Read the model definition and answer for the solid it produces. Units are mm, in the model's axes. Face numbers are marked on the shaded views. A direction names the side the tool comes from. Coordinates: 2 decimals unless noted, no trailing zeros. Write each loop counter-clockwise with the first axis right and the second up, starting at its lowest first coordinate (ties: lowest second). Pieces come first, ordered by that corner, then holes. Notation, with made-up numbers: (41.5, 55.25) -> (84.5, 55.25) arc R25 ccw to (84.5, 88.25) -> close; hole circle Ø8 at (62.25, 55). An arc over 180 degrees is marked (long way). Answer as a JSON object with one key per item and string values. Group by question number.
(1) Find section D-D (y = 38.1). Give the vertices of the cut face in (x, z).
(2) Find section B-B (x = 42.5). Give the vertices of the cut face in (y, z), then the cut area to 3 significant figures.
(3) For a pull along Z with two mould halves and no side action, classify the marked faces 1, 2, 3 and 4 as +Z half, -Z half, draft (parallel to the pull), parting line (faces both ways), or undercut.
(4) Straight lines are drawn through the part: L1, parallel to Y at x = 72, z = -25; L2, parallel to Z at x = 69, y = 38; L3, parallel to Y at x = 38.5, z = -17. For each, find the intervals that lie inside material, in ascending order.
(5) Which of the six approach directions +Z, -Z, +X, -X, +Y, -Y give full straight-line access (tool end or side, diameter ignored) to the marked faces 5 and 6?
(6) Find section C-C (z = -28). Give the vertices of the cut face in (x, y), then the cut area to 3 significant figures.
(7) Flat-ended cylindrical pins translate along their axes: P1, Ø12.5, axis at x = 28, z = -26.5, coming from the +Y side; P2, Ø23, axis at y = 38.1, z = -25.4, coming from the +X side. Find the tip coordinate at first contact, or state that the pin passes through.
(8) Find section A-A (y = 54). Give the vertices of the cut face in (x, z).
from build123d import *

# Parameters (mm, degrees)
SKETCH1_W           = 76.2
SKETCH1_H           = 50.8
BOSS_EXTRUDE1_DEPTH = 76.2
SKETCH2_W           = 38.1
SKETCH2_H           = 25.4
CUT_EXTRUDE1_DEPTH  = 25.4
SKETCH3_R           = 12.7
CUT_EXTRUDE3_DEPTH  = 12.7


with BuildPart() as part:
    # Sketch1 → Boss-Extrude1 (new body)
    with BuildSketch(Plane(origin=(0, 0, 0), x_dir=(1, 0, 0), z_dir=(0, 1, 0))):
        with Locations((38.1, 25.4)):
            Rectangle(SKETCH1_W, SKETCH1_H)
    extrude(amount=BOSS_EXTRUDE1_DEPTH)

    # Sketch2 → Cut-Extrude1 (cut)
    with BuildSketch(Plane(origin=(0, 76.2, 0), x_dir=(1, 0, 0), z_dir=(0, 1, 0))):
        with Locations((31.75, 25.4)):
            Rectangle(SKETCH2_W, SKETCH2_H)
    extrude(amount=-CUT_EXTRUDE1_DEPTH, mode=Mode.SUBTRACT)

    # Sketch3 → Cut-Extrude3 (cut)
    with BuildSketch(Plane(origin=(76.2, 0, 0), x_dir=(0, 0, -1), z_dir=(1, 0, 0))):
        with Locations((25.4, 38.1)):
            Circle(SKETCH3_R)
    extrude(amount=-CUT_EXTRUDE3_DEPTH, mode=Mode.SUBTRACT)


solid = part.part
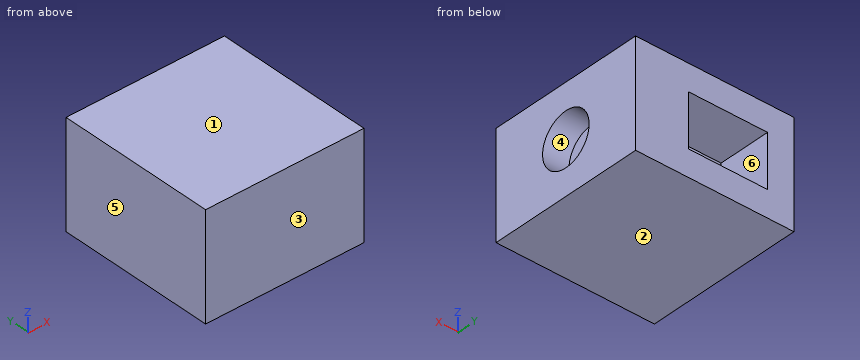
Results below:
{
 "1": {"outline": "(0, -50.8) -> (76.2, -50.8) -> (76.2, -38.1) -> (63.5, -38.1) -> (63.5, -12.7) -> (76.2, -12.7) -> (76.2, 0) -> (0, 0) -> close"},
 "2": {"outline": "(0, -50.8) -> (76.2, -50.8) -> (76.2, -38.1) -> (50.8, -38.1) -> (50.8, -12.7) -> (76.2, -12.7) -> (76.2, 0) -> (0, 0) -> close", "area": "3,230 mm2"},
 "3": {"face 1": "+Z half", "face 2": "-Z half", "face 3": "draft", "face 4": "undercut"},
 "4": {"L1": "y = 0 to 25.41, 50.79 to 76.2", "L2": "z = -50.8 to -38.1, -12.7 to 0", "L3": "y = 0 to 50.8"},
 "5": {"face 5": "+Z, -Z, -X, +Y, -Y", "face 6": "+Y"},
 "6": {"outline": "(0, 0) -> (76.2, 0) -> (76.2, 25.67) -> (63.5, 25.67) -> (63.5, 50.53) -> (76.2, 50.53) -> (76.2, 76.2) -> (50.8, 76.2) -> (50.8, 50.8) -> (12.7, 50.8) -> (12.7, 76.2) -> (0, 76.2) -> close", "area": "4,520 mm2"},
 "7": {"P1": "stops at y = 50.8", "P2": "stops at x = 63.5"},
 "8": {"outline": "(0, -50.8) -> (76.2, -50.8) -> (76.2, 0) -> (0, 0) -> close; hole (12.7, -38.1) -> (50.8, -38.1) -> (50.8, -12.7) -> (12.7, -12.7) -> close"}
}
